from build123d import *

# Parameters (mm, degrees)
BOSS_EXTRUDE1_DEPTH  = 5
CUT_EXTRUDE1_DEPTH   = 6
FILLET1_R            = 10
M6_CLEARANCE_HOLE1_D = 6.6
FILLET2_R            = 0.5
SKETCH5_R            = 1
CUT_EXTRUDE2_DEPTH   = 6
FILLET3_R            = 2
CUT_EXTRUDE3_DEPTH   = 2
FILLET4_R            = 2


with BuildPart() as part:
    # Sketch1 → Boss-Extrude1 (new body)
    with BuildSketch(Plane(origin=(0, 0, 0), x_dir=(1, 0, 0), z_dir=(0, 1, 0))):
        with BuildLine():
            Line((-25.590540252, 6.833634535), (-14.025260906, 12.064081255))
            ThreePointArc((-14.025260906, 12.064081255), (0, 18.5), (14.025260906, 12.064081255))
            Line((14.025260906, 12.064081255), (25.590540252, 6.833634535))
            ThreePointArc((25.590540252, 6.833634535), (29.83151618, -1.580781609), (22.5, -7.5))
            Line((22.5, -7.5), (-22.5, -7.5))
            ThreePointArc((-22.5, -7.5), (-29.83151618, -1.580781609), (-25.590540252, 6.833634535))
        make_face()
    extrude(amount=BOSS_EXTRUDE1_DEPTH)

    # Sketch2 → Cut-Extrude1 (cut, through all)
    with BuildSketch(Plane(origin=(0, 5, 0), x_dir=(1, 0, 0), z_dir=(0, 1, 0))):
        with BuildLine():
            Line((10, -7.5), (10, 1.661480829))
            Line((10, 1.661480829), (5.765369152, 1.661480829))
            ThreePointArc((5.765369152, 1.661480829), (0, 6), (-5.765369152, 1.661480829))
            Line((-5.765369152, 1.661480829), (-10, 1.661480829))
            Line((-10, 1.661480829), (-10, -7.5))
            Line((-10, -7.5), (10, -7.5))
        make_face()
    extrude(amount=-CUT_EXTRUDE1_DEPTH, mode=Mode.SUBTRACT)

    # Fillet1
    fillet1_edges = [part.edges().sort_by_distance(p)[0] for p in [
        (-14.025260906, 2.5, -12.064081255),
        (14.025260906, 2.5, -12.064081255),
    ]]
    fillet(fillet1_edges, radius=FILLET1_R)

    # M6 Clearance Hole1 (through all)
    with Locations(Plane(origin=(0, 5, 0), x_dir=(1, 0, 0), z_dir=(0, 1, 0))):
        with Locations((-22.5, 0), (22.5, 0)):
            Hole(M6_CLEARANCE_HOLE1_D / 2)

    # Fillet2
    fillet2_edges = [part.edges().sort_by_distance(p)[0] for p in [
        (-5.765369152, 2.5, -1.661480829),
        (5.765369152, 2.5, -1.661480829),
    ]]
    fillet(fillet2_edges, radius=FILLET2_R)

    # Sketch5 → Cut-Extrude2 (cut, through all)
    with BuildSketch(Plane(origin=(0, 5, 0), x_dir=(1, 0, 0), z_dir=(0, 1, 0))):
        with Locations((-10, 1.661480829)):
            Circle(SKETCH5_R)
        with Locations((10, 1.661480829)):
            Circle(SKETCH5_R)
    extrude(amount=-CUT_EXTRUDE2_DEPTH, mode=Mode.SUBTRACT)

    # Fillet3
    fillet3_edges = [part.edges().sort_by_distance(p)[0] for p in [
        (10, 2.5, 7.5),
        (-10, 2.5, 7.5),
    ]]
    fillet(fillet3_edges, radius=FILLET3_R)

    # Sketch6 → Cut-Extrude3 (cut)
    with BuildSketch(Plane.XZ):
        with BuildLine():
            Line((-13.5, 0), (-13.5, 12))
            ThreePointArc((-13.5, 12), (0, 25.5), (13.5, 12))
            Line((13.5, 12), (13.5, 0))
            ThreePointArc((13.5, 0), (0, -13.5), (-13.5, 0))
        make_face()
    extrude(amount=-CUT_EXTRUDE3_DEPTH, mode=Mode.SUBTRACT)

    # Fillet4
    fillet4_edges = [part.edges().sort_by_distance(p)[0] for p in [
        (-13.5, 1, 7.5),
        (13.5, 1, 7.5),
    ]]
    fillet(fillet4_edges, radius=FILLET4_R)


solid = part.part
Work out the finished part from the listing and answer in its coordinate system (mm). A direction names the side the tool comes from. Give positions to 0.01 mm unless a question says otherwise; leave off trailing zeros. Order: outer loops, then holes, each group sorted by start corner. A loop starts at its lowest first (then second) coordinate and runs counter-clockwise, first axis right, second up. Notation, with made-up numbers: M 69.25,-31.75 L 99.25,-31.75 A10 cw 99.25,-16.75 Z; hole C -3,-21 d7. An arc over 180 degrees is marked long. Return JSON: item names as keys, results as strings.
Q1. Find section B-B, the plane x = -23.5. Write down the section's boundary in (y, z).
Answer below:
{"outline": "M 0,-7.78 L 5,-7.78 L 5,-3.14 L 0,-3.14 Z; M 0,3.14 L 5,3.14 L 5,7.43 L 0,7.43 Z"}
Q2. Find section C-C, the plane y = 1.4. Write down the section's boundary in (x, z), and give its area (3 significant figures).
Answer below:
{"outline": "M -25.59,-6.83 L -15.82,-11.25 A10 cw -12.94,-13.22 A18.5 ccw 12.94,-13.22 A10 cw 15.82,-11.25 L 25.59,-6.83 A7.5 ccw 22.5,7.5 L 15.5,7.5 A2 ccw 13.5,5.5 L 13.5,0 A13.5 cw -13.5,0 L -13.5,5.5 A2 ccw -15.5,7.5 L -22.5,7.5 A7.5 ccw Z; hole C -22.5,0 d6.6; hole C 22.5,0 d6.6", "area": "593 mm^2"}
Q3. Which of the six approach directions +Z, -Z, +X, -X, +Y, -Y give full straight-line access (tool end or side, diameter ignored) to faces 4 (the face through (-8, 4, -1.661)), 5 (the face through (-13.5, 1, 3)), 6 (the face through (-25.55, 2.47, 1.26))?
Answer below:
{"face 4": "+Z, +Y, -Y", "face 5": "+Z, -Y", "face 6": "+Y, -Y"}
Q4. Find section D-D, the plane z = -12.25. Write down the section's boundary in (x, y), and give its area (3 significant figures).
Answer below:
{"outline": "M -14.09,0 L -5.67,0 L -5.67,2 L 5.67,2 L 5.67,0 L 14.09,0 L 14.09,5 L -14.09,5 Z", "area": "118 mm^2"}
Q5. The mould has two halves that part along X. Classify faces 1 (the face through (-18, 2, 7.5)), 2 (the face through (20.635, 2.465, -9.075)), 3 (the face through (10, 4, 2)): pulls with the +X half, pulls with the -X half, needs draft (parallel to the pull), parting line crosses it, or undercut.
Answer below:
{"face 1": "needs draft", "face 2": "pulls with the +X half", "face 3": "undercut"}
Q6. Find section A-A, the plane y = 3.9. Write down the section's boundary in (x, z), and give its area (3 significant figures).
Answer below:
{"outline": "M -25.59,-6.83 L -15.82,-11.25 A10 cw -12.94,-13.22 A18.5 ccw 12.94,-13.22 A10 cw 15.82,-11.25 L 25.59,-6.83 A7.5 ccw 22.5,7.5 L 12,7.5 A2 ccw 10,5.5 L 10,-0.66 A1 cw long 9,-1.66 L 6.13,-1.66 A0.5 ccw 5.66,-2 A6 cw -5.66,-2 A0.5 ccw -6.13,-1.66 L -9,-1.66 A1 cw long -10,-0.66 L -10,5.5 A2 ccw -12,7.5 L -22.5,7.5 A7.5 ccw Z; hole C -22.5,0 d6.6; hole C 22.5,0 d6.6", "area": "857 mm^2"}
Q7. Find the intervals of material crossed by line 1 along X through (y, z) = (1.55, -1); line 2 along X through (y, z) = (3.35, -2.75); line 3 along Y through (x, z) = (0, -6.75), in increasing order. Write a range as [from, to].
Answer below:
{"line 1": "x = [-29.93, -25.64], [-19.36, -13.46], [13.46, 19.36], [25.64, 29.93]", "line 2": "x = [-29.48, -24.32], [-20.68, -5.33], [5.33, 20.68], [24.32, 29.48]", "line 3": "y = [2, 5]"}
Q8. Each of these flat-tipped pins is pushed along its axis until it touches: pin 1 (4 mm diameter, centred on x = 19.5, z = -0.5, fed in from -Y); pin 2 (1.4 mm diameter, centred on x = -7, y = 3.5, fed in from +Z); pin 3 (1.5 mm diameter, centred on y = 3, z = 2, fed in from -X); pin 4 (3 mm diameter, centred on y = 0.5, z = 3.5, fed in from -X). Where does it stop, or does it pass through?
Answer below:
{"pin 1": "stops at y = 0", "pin 2": "stops at z = -1.66", "pin 3": "stops at x = -29.9", "pin 4": "stops at x = -29.73"}
